Read the model definition and answer for the solid it produces. Units are mm, in the model's axes. Face numbers are marked on the shaded views. A direction names the side the tool comes from. Give positions to 0.01 mm unless a question says otherwise; leave off trailing zeros. Order: outer loops, then holes, each group sorted by start corner. A loop starts at its lowest first (then second) coordinate and runs counter-clockwise, first axis right, second up.
Item 1: A cutting plane is placed at A-A (z = 25). Write down the section's boundary in (x, y), plus the area to 3 significant figures.
Item 2: Which of the six approach directions +Z, -Z, +X, -X, +Y, -Y give full straight-line access (tool end or side, diameter ignored) to the marked faces 1 and 2?
Item 3: Given pin 1 Ø3 at (y, z) = (39.87, 40.5) entering from +X; pin 2 Ø2.5 at (x, y) = (31.5, -1.5) entering from -Z; pin 3 Ø3 at (y, z) = (9.5, 37.5) entering from +X; pin 4 Ø24.5 at (x, z) = (21, 33) entering from +Y, each flat-ended and moving along its own axis, determine where each tip first touches the part or whether it passes through.
Item 4: A cutting plane is placed at B-B (x = 13.5). Write down the section's boundary in (y, z).
Item 5: Find the intervals of material crossed by line 1 along Y through (x, z) = (-2.1, 40.5); line 2 along Y through (x, z) = (8.5, 15), in increasing order.
Item 6: A cutting plane is placed at D-D (z = 10). Write down the section's boundary in (x, y), plus the area to 3 significant figures.
Item 7: A cutting plane is placed at C-C (y = 28.5). Write down the section's boundary in (x, z), plus the area to 3 significant figures.
from build123d import *

# Parameters (mm, degrees)
SM_BASE_FLANGE_1_DEPTH = 50
SKETCH_7_R             = 11.05
SKETCH_7_R_2           = 1.75
CUT_EXTRUDE_1_DEPTH    = 10
CUT_EXTRUDE_2_DEPTH    = 10


# Sheet-metal steps are written as plain solids
with BuildPart() as part:
    # Sketch 2 → 基体-法兰1 (new body)
    with BuildSketch(Plane.XY):
        with BuildLine():
            Line((50, 0), (0.7366, 0))
            ThreePointArc((0.7366, 0), (0.215745145, 0.215745145), (0, 0.7366))
            Line((0, 0.7366), (0, 48))
            Line((0, 48), (-3, 48))
            Line((-3, 48), (-3, 0.7366))
            ThreePointArc((-3, 0.7366), (-1.905575199, -1.905575199), (0.7366, -3))
            Line((0.7366, -3), (50, -3))
            Line((50, -3), (50, 0))
        make_face()
    extrude(amount=SM_BASE_FLANGE_1_DEPTH)

    # 草图7 → 切除-拉伸1 (cut)
    with BuildSketch(Plane(origin=(0, 0, 0), x_dir=(0, 0, -1), z_dir=(1, 0, 0))):
        with Locations((-25, 24.3683)):
            Circle(SKETCH_7_R)
        with Locations((-40.5, 39.8683)):
            Circle(SKETCH_7_R_2)
        with Locations((-9.5, 39.8683)):
            Circle(SKETCH_7_R_2)
        with Locations((-40.5, 8.8683)):
            Circle(SKETCH_7_R_2)
        with Locations((-9.5, 8.8683)):
            Circle(SKETCH_7_R_2)
    extrude(amount=-CUT_EXTRUDE_1_DEPTH, mode=Mode.SUBTRACT)

    # 草图8 → 切除-拉伸2 (cut)
    with BuildSketch(Plane(origin=(0, 0, 0), x_dir=(1, 0, 0), z_dir=(0, 1, 0))):
        with BuildLine():
            Line((9, -12.1), (39, -12.1))
            ThreePointArc((39, -12.1), (41.1, -10), (39, -7.9))
            Line((39, -7.9), (9, -7.9))
            ThreePointArc((9, -7.9), (6.9, -10), (9, -12.1))
        make_face()
        with BuildLine():
            Line((9, -42.1), (39, -42.1))
            ThreePointArc((39, -42.1), (41.1, -40), (39, -37.9))
            Line((39, -37.9), (9, -37.9))
            ThreePointArc((9, -37.9), (6.9, -40), (9, -42.1))
        make_face()
    extrude(amount=-CUT_EXTRUDE_2_DEPTH, mode=Mode.SUBTRACT)


solid = part.part
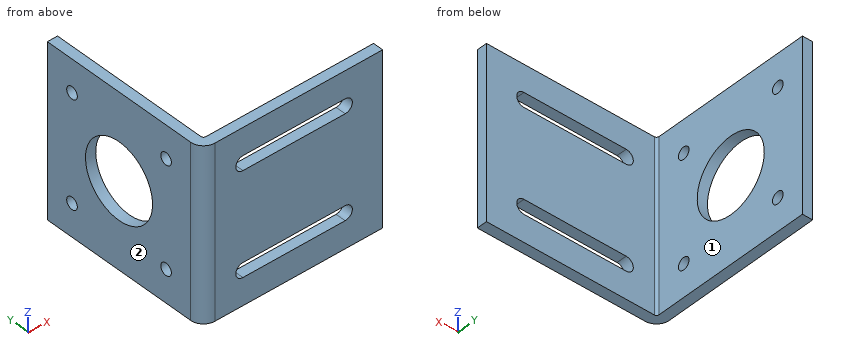
Response values:
1. outline: (-3, 0.74) arc R3.74 ccw to (0.74, -3) - (50, -3) - (50, 0) - (0.74, 0) arc R0.74 cw to (0, 0.74) - (0, 13.32) - (-3, 13.32) - close; (-3, 35.42) - (0, 35.42) - (0, 48) - (-3, 48) - close
1. area: 234 mm2
2. face 1: +Z, -Z, +X, +Y
2. face 2: +Z, -Z, -X, +Y, -Y
3. pin 1: passes through
3. pin 2: stops at z = 0
3. pin 3: stops at x = 0
3. pin 4: stops at y = 0
4. outline: (-3, 0) - (0, 0) - (0, 7.9) - (-3, 7.9) - close; (-3, 12.1) - (0, 12.1) - (0, 37.9) - (-3, 37.9) - close; (-3, 42.1) - (0, 42.1) - (0, 50) - (-3, 50) - close
5. line 1: y = -1.7 to 7.12, 10.62 to 38.12, 41.62 to 48
5. line 2: y = -3 to 0
6. outline: (-3, 0.74) arc R3.74 ccw to (0.74, -3) - (6.9, -3) - (6.9, 0) - (0.74, 0) arc R0.74 cw to (0, 0.74) - (0, 7.19) - (-3, 7.19) - close; (-3, 10.55) - (0, 10.55) - (0, 38.19) - (-3, 38.19) - close; (-3, 41.55) - (0, 41.55) - (0, 48) - (-3, 48) - close; (41.1, -3) - (50, -3) - (50, 0) - (41.1, 0) - close
6. area: 177 mm2
7. outline: (-3, 0) - (0, 0) - (0, 14.75) - (-3, 14.75) - close; (-3, 35.25) - (0, 35.25) - (0, 50) - (-3, 50) - close
7. area: 88.5 mm2
